from build123d import *

# Parameters (mm, degrees)
SKETCH1_W           = 300
SKETCH1_H           = 300
BOSS_EXTRUDE1_DEPTH = 300
SKETCH3_R           = 79.895545122
CUT_EXTRUDE1_DEPTH  = 100
SKETCH8_R           = 50
CUT_EXTRUDE3_DEPTH  = 100
SKETCH9_W           = 73.610989956
SKETCH9_H           = 275.007350114
CUT_EXTRUDE4_DEPTH  = 80
SKETCH11_W          = 132.256824298
SKETCH11_H          = 300
CUT_EXTRUDE6_DEPTH  = 40


with BuildPart() as part:
    # Sketch1 → Boss-Extrude1 (new body)
    with BuildSketch(Plane(origin=(0, 0, 0), x_dir=(1, 0, 0), z_dir=(0, 1, 0))):
        Rectangle(SKETCH1_W, SKETCH1_H)
    extrude(amount=BOSS_EXTRUDE1_DEPTH)

    # Sketch3 → Cut-Extrude1 (cut)
    with BuildSketch(Plane(origin=(0, 0, 0), x_dir=(1, 0, 0), z_dir=(0, 1, 0))):
        with Locations(Location((-63.272367771, -59.757236228, 0), (0, 0, 270))):
            Circle(SKETCH3_R)
    extrude(amount=CUT_EXTRUDE1_DEPTH, mode=Mode.SUBTRACT)

    # Sketch8 → Cut-Extrude3 (cut)
    with BuildSketch(Plane.XZ):
        with Locations(Location((-70.716175744, -86.224109021, 0), (0, 0, 270))):
            Circle(SKETCH8_R)
    extrude(amount=-CUT_EXTRUDE3_DEPTH, mode=Mode.SUBTRACT)

    # Sketch9 → Cut-Extrude4 (cut)
    with BuildSketch(Plane.XZ):
        with Locations((91.393420113, 0)):
            Rectangle(SKETCH9_W, SKETCH9_H)
    extrude(amount=-CUT_EXTRUDE4_DEPTH, mode=Mode.SUBTRACT)

    # Sketch11 → Cut-Extrude6 (cut)
    with BuildSketch(Plane(origin=(0, 300, 0), x_dir=(1, 0, 0), z_dir=(0, 1, 0))):
        Rectangle(SKETCH11_W, SKETCH11_H)
    extrude(amount=-CUT_EXTRUDE6_DEPTH, mode=Mode.SUBTRACT)


solid = part.part
Design review of the part built by this model. Coordinates are the model's own, in mm. A direction names the side the tool comes from. Coordinates: 2 decimals unless noted, no trailing zeros. Order: outer loops, then holes, each group sorted by start corner. A loop starts at its lowest first (then second) coordinate and runs counter-clockwise, first axis right, second up. Notation, with made-up numbers: (15.25, -25) -> (62.25, -25) arc R16 ccw to (62.25, -14) -> close; hole circle Ø5 at (62.25, -29.75). An arc over 180 degrees is marked (long way). One line per item, written item: value.
1) To check wall thickness, follow probe 1 along X at (y, z) = (50.5, -87); probe 2 along Z at (x, y) = (-107, 98); probe 3 along Z at (x, y) = (-87, 68). State the ranges of each line that lie inside material, in increasing order. Write a range as [from, to].
Output values:
probe 1: x = [-150, -120.71], [-20.72, 54.59], [128.2, 150]
probe 2: z = [-150, -120.63], [-51.82, -7.11], [126.62, 150]
probe 3: z = [-150, -133.5], [-38.95, -16.53], [136.05, 150]
2) We need section B-B, the plane y = 86.5. Give the boundary of the cut face in (x, z), then the cut area to 3 significant figures.
Output values:
outline: (-150, -150) -> (150, -150) -> (150, 150) -> (-150, 150) -> close; hole circle Ø159.79 at (-63.27, 59.76); hole circle Ø100 at (-70.72, -86.22)
area: 62,100 mm2
3) Draft analysis for pull direction X (two halves, no side actions). For faces 4 (the face through (-150, 148, 2)), 5 (the face through (107, 300, -2)), 6 (the face through (91, 39, -137.504)), state which applies: +X half, -X half, draft (parallel to the pull), parting line (faces both ways), or undercut.
Output values:
face 4: -X half
face 5: draft
face 6: undercut
4) We need section A-A, the plane x = 80. Give the boundary of the cut face in (y, z).
Output values:
outline: (0, -150) -> (300, -150) -> (300, 150) -> (0, 150) -> (0, 137.5) -> (80, 137.5) -> (80, -137.5) -> (0, -137.5) -> close
5) We need section C-C, the plane z = 63. Give the boundary of the cut face in (x, y).
Output values:
outline: (-150, 0) -> (-143.1, 0) -> (-143.1, 100) -> (16.56, 100) -> (16.56, 0) -> (54.59, 0) -> (54.59, 80) -> (128.2, 80) -> (128.2, 0) -> (150, 0) -> (150, 300) -> (66.13, 300) -> (66.13, 260) -> (-66.13, 260) -> (-66.13, 300) -> (-150, 300) -> close
6) Machinability: for faces 1 (the face through (-66.128, 280, 2)), 2 (the face through (-2, 148, -150)), 3 (the face through (-70, 100, -86)), which of the approach directions +Z, -Z, +X, -X, +Y, -Y give a long, thin tool a straight path to every point of the face, cutting with its end or side? Answer none if there is none.
Output values:
face 1: +Z, -Z, +Y
face 2: -Z, +X, -X, +Y, -Y
face 3: -Y
7) We need section D-D, the plane y = 48. Give the boundary of the cut face in (x, z), then the cut area to 3 significant figures.
Output values:
outline: (-150, -150) -> (150, -150) -> (150, 150) -> (-150, 150) -> close; hole circle Ø159.79 at (-63.27, 59.76); hole circle Ø100 at (-70.72, -86.22); hole (54.59, -137.5) -> (128.2, -137.5) -> (128.2, 137.5) -> (54.59, 137.5) -> close
area: 41,800 mm2
